Read the model definition and answer for the solid it produces. Units are mm, in the model's axes. Give positions to 0.01 mm unless a question says otherwise; leave off trailing zeros. Order: outer loops, then holes, each group sorted by start corner. A loop starts at its lowest first (then second) coordinate and runs counter-clockwise, first axis right, second up. Notation, with made-up numbers: (84.5, -21.5) -> (123.5, -21.5) arc R27 cw to (123.5, -5.5) -> close; hole circle Ø8 at (7.25, 66). An arc over 180 degrees is marked (long way). Use one line per item in the form item = value.
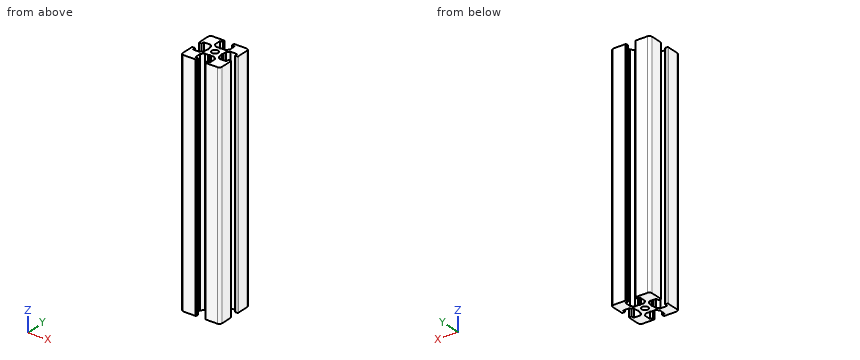
Autodesk Inventor part; units mm, degrees
ref_plane "YZ Plane" through (0, 0, 0) normal (1, 0, 0) x (0, 1, 0)
ref_plane "XZ Plane" through (0, 0, 0) normal (0, 1, 0) x (-1, 0, 0)
ref_plane "XY Plane" through (0, 0, 0) normal (0, 0, 1) x (1, 0, 0)
sketch "Sketch_1" plane through (0, 0, 0) normal (0, 0, 1) x (1, 0, 0)
  line L0 (-7.5, 6.5) -> (-7.5, 2)
  arc A0 (-7.5, 2) -> (-7.2, 1.7) centre (-7.2, 2) ccw
  line L1 (-7.2, 1.7) -> (-6.4, 1.7)
  line L2 (-6.4, 1.7) -> (-6.4, 2.85)
  line L3 (-6.4, 2.85) -> (-3.8, 2.85)
  line L4 (-3.8, 2.85) -> (-2.8, 1.85)
  line L5 (-2.8, 1.85) -> (-2.8, 0.5196)
  line L6 (-2.8, 0.5196) -> (-2.5, 0)
  line L7 (-2.5, 0) -> (-2.8, -0.5196)
  line L8 (-2.8, -0.5196) -> (-2.8, -1.85)
  line L9 (-2.8, -1.85) -> (-3.8, -2.85)
  line L10 (-3.8, -2.85) -> (-6.4, -2.85)
  line L11 (-6.4, -2.85) -> (-6.4, -1.7)
  line L12 (-6.4, -1.7) -> (-7.2, -1.7)
  arc A1 (-7.2, -1.7) -> (-7.5, -2) centre (-7.2, -2) ccw
  line L13 (-7.5, -2) -> (-7.5, -6.5)
  arc A2 (-7.5, -6.5) -> (-6.5, -7.5) centre (-6.5, -6.5) ccw
  line L14 (-6.5, -7.5) -> (-2, -7.5)
  arc A3 (-2, -7.5) -> (-1.7, -7.2) centre (-2, -7.2) ccw
  line L15 (-1.7, -7.2) -> (-1.7, -6.4)
  line L16 (-1.7, -6.4) -> (-2.85, -6.4)
  line L17 (-2.85, -6.4) -> (-2.85, -3.8)
  line L18 (-2.85, -3.8) -> (-1.85, -2.8)
  line L19 (-1.85, -2.8) -> (-0.5196, -2.8)
  line L20 (-0.5196, -2.8) -> (0, -2.5)
  line L21 (0, -2.5) -> (0.5196, -2.8)
  line L22 (0.5196, -2.8) -> (1.85, -2.8)
  line L23 (1.85, -2.8) -> (2.85, -3.8)
  line L24 (2.85, -3.8) -> (2.85, -6.4)
  line L25 (2.85, -6.4) -> (1.7, -6.4)
  line L26 (1.7, -6.4) -> (1.7, -7.2)
  arc A4 (1.7, -7.2) -> (2, -7.5) centre (2, -7.2) ccw
  line L27 (2, -7.5) -> (6.5, -7.5)
  arc A5 (6.5, -7.5) -> (7.5, -6.5) centre (6.5, -6.5) ccw
  line L28 (7.5, -6.5) -> (7.5, -2)
  arc A6 (7.5, -2) -> (7.2, -1.7) centre (7.2, -2) ccw
  line L29 (7.2, -1.7) -> (6.4, -1.7)
  line L30 (6.4, -1.7) -> (6.4, -2.85)
  line L31 (6.4, -2.85) -> (3.8, -2.85)
  line L32 (3.8, -2.85) -> (2.8, -1.85)
  line L33 (2.8, -1.85) -> (2.8, -0.5196)
  line L34 (2.8, -0.5196) -> (2.5, 0)
  line L35 (2.5, 0) -> (2.8, 0.5196)
  line L36 (2.8, 0.5196) -> (2.8, 1.85)
  line L37 (2.8, 1.85) -> (3.8, 2.85)
  line L38 (3.8, 2.85) -> (6.4, 2.85)
  line L39 (6.4, 2.85) -> (6.4, 1.7)
  line L40 (6.4, 1.7) -> (7.2, 1.7)
  arc A7 (7.2, 1.7) -> (7.5, 2) centre (7.2, 2) ccw
  line L41 (7.5, 2) -> (7.5, 6.5)
  arc A8 (7.5, 6.5) -> (6.5, 7.5) centre (6.5, 6.5) ccw
  line L42 (6.5, 7.5) -> (2, 7.5)
  arc A9 (2, 7.5) -> (1.7, 7.2) centre (2, 7.2) ccw
  line L43 (1.7, 7.2) -> (1.7, 6.4)
  line L44 (1.7, 6.4) -> (2.85, 6.4)
  line L45 (2.85, 6.4) -> (2.85, 3.8)
  line L46 (2.85, 3.8) -> (1.85, 2.8)
  line L47 (1.85, 2.8) -> (0.5196, 2.8)
  line L48 (0.5196, 2.8) -> (0, 2.5)
  line L49 (0, 2.5) -> (-0.5196, 2.8)
  line L50 (-0.5196, 2.8) -> (-1.85, 2.8)
  line L51 (-1.85, 2.8) -> (-2.85, 3.8)
  line L52 (-2.85, 3.8) -> (-2.85, 6.4)
  line L53 (-2.85, 6.4) -> (-1.7, 6.4)
  line L54 (-1.7, 6.4) -> (-1.7, 7.2)
  arc A10 (-1.7, 7.2) -> (-2, 7.5) centre (-2, 7.2) ccw
  line L55 (-2, 7.5) -> (-6.5, 7.5)
  arc A11 (-6.5, 7.5) -> (-7.5, 6.5) centre (-6.5, 6.5) ccw
  circle A12 centre (0, 0) radius 1.25
extrude "Extrusion1" add sketch "Sketch_1" along normal blind 90
properties part number "HFS3-1515-90"
Item 1: Straight lines are drawn through the part: L1, parallel to Y at x = 0, z = 45.5; L2, parallel to X at y = -4, z = 63.5. For each, find the intervals that lie inside material, in ascending order. Write a range as from..to.
Checks:
L1 = -2.5..-1.25, 1.25..2.5
L2 = -7.5..-2.85, 2.85..7.5
Item 2: Given pin 1 Ø1.1 at (x, z) = (-1, 51) entering from +Y; pin 2 Ø0.7 at (y, z) = (1.5, 61.5) entering from -X; pin 3 Ø1.1 at (x, z) = (1, 60) entering from -Y, each flat-ended and moving along its own axis, determine where each tip first touches the part or whether it passes through.
Checks:
pin_1 = 2.8
pin_2 = -7.46
pin_3 = -2.8
Item 3: The part is cut by section A-A on x = 4.75. Give the vertices of the cut face in (y, z), and give its area (3 significant figures).
Checks:
outline = (-7.5, 0) -> (-2.85, 0) -> (-2.85, 90) -> (-7.5, 90) -> close; (2.85, 0) -> (7.5, 0) -> (7.5, 90) -> (2.85, 90) -> close
area = 837 mm²
